Here's the drawing with two shaded views (mm, measured from the low corner). I have some questions. Coordinates: 2 decimals unless noted, no trailing zeros. Order: outer loops, then holes, each group sorted by start corner. A loop starts at its lowest first (then second) coordinate and runs counter-clockwise, first axis right, second up. Notation, with made-up numbers: (59, 37.5) - (112, 37.5) arc R19 ccw to (112, 60.5) - close; hole circle Ø5 at (68.5, 30.5). An arc over 180 degrees is marked (long way). Answer as a JSON object with one key per item and string values. Group by question number.
(1) Will these pins go through, and if not, where does the flat tip stop? P1, Ø1.6, axis at y = 1, z = 34, coming from the +X side (3 decimals); P2, Ø1.6, axis at x = 1, y = 2, coming from the +Z side; P3, Ø1.6, axis at y = 1.5, z = 6, coming from the -X side (3 decimals).
(2) Imagine slicing it at A-A, the plane y = 0.95. Write out the boundary of the cut face in (x, z) (3 decimals).
(3) Please list where these lines run through material, in increasing order: probe 1 along X at (y, z) = (0.2, 34.5) (3 decimals); probe 2 along Z at (x, y) = (53.5, 1.8); probe 3 along X at (y, z) = (2.45, 27) (3 decimals).
(4) Imagine slicing it at B-B, the plane z = 4. Write out the boundary of the cut face in (x, y) (3 decimals), and give its area (3 significant figures).
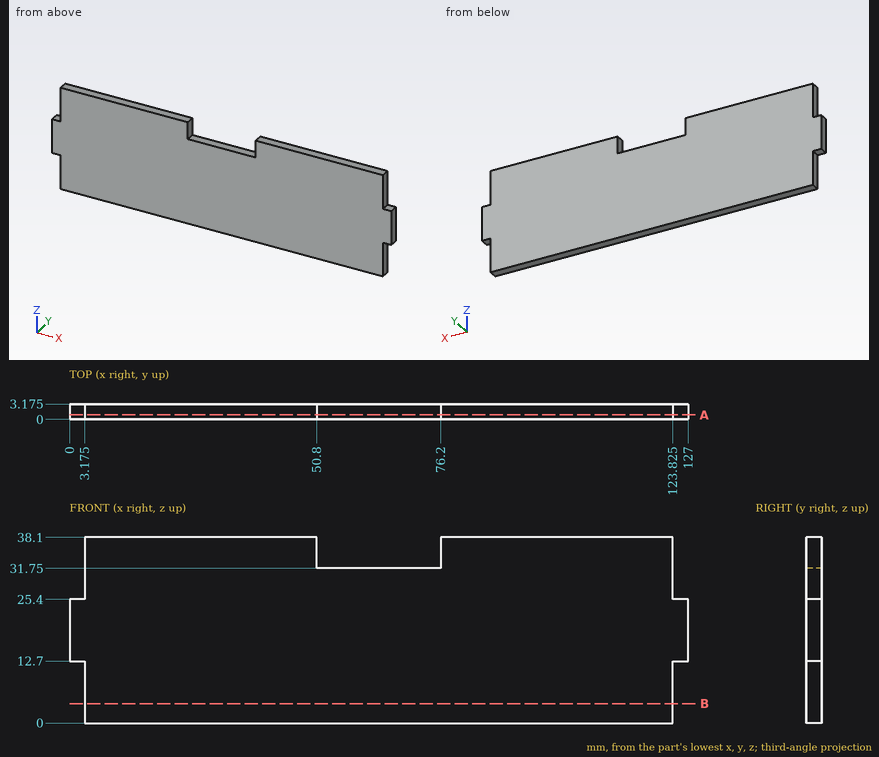
Result set:
{
 "1": {"P1": "stops at x = 123.825", "P2": "stops at z = 25.4", "P3": "stops at x = 3.175"},
 "2": {"outline": "(0, 12.7) - (3.175, 12.7) - (3.175, 0) - (123.825, 0) - (123.825, 12.7) - (127, 12.7) - (127, 25.4) - (123.825, 25.4) - (123.825, 38.1) - (76.2, 38.1) - (76.2, 31.75) - (50.8, 31.75) - (50.8, 38.1) - (3.175, 38.1) - (3.175, 25.4) - (0, 25.4) - close"},
 "3": {"probe 1": "x = 3.175 to 50.8, 76.2 to 123.825", "probe 2": "z = 0 to 31.75", "probe 3": "x = 3.175 to 123.825"},
 "4": {"outline": "(3.175, 0) - (123.825, 0) - (123.825, 3.175) - (3.175, 3.175) - close", "area": "383 mm^2"}
}
